Verification items for the finished model (mm, model axes). Coordinates: 2 decimals unless noted, no trailing zeros. Use CSV: the item, a comma, the result in double quotes. Start each with the question number.
```python
from build123d import *

# Parameters (mm, degrees)
BOSS_EXTRUDE2_DEPTH = 9.5
FILLET1_R           = 0.5


with BuildPart() as part:
    # Sketch2 → Boss-Extrude2 (new body, symmetric)
    with BuildSketch(Plane(origin=(0, 0, 0), x_dir=(0, 0, -1), z_dir=(1, 0, 0))):
        with BuildLine():
            Line((0, 12), (0, -12))
            ThreePointArc((0, -12), (-5.710285596, -12.497714363), (-11, -10.29))
            ThreePointArc((-11, -10.29), (-9.540341867, 0), (-11, 10.29))
            ThreePointArc((-11, 10.29), (-5.710285596, 12.497714363), (0, 12))
        make_face()
    extrude(amount=BOSS_EXTRUDE2_DEPTH, both=True)

    # Fillet1
    fillet1_edges = [part.edges().sort_by_distance(p)[0] for p in [
        (9.5, 12.497714363, 5.710285596),
        (9.5, 0, 9.540341867),
        (9.5, -12.497714363, 5.710285596),
        (-9.5, 0, 9.540341867),
        (-9.5, 12.497714363, 5.710285596),
        (-9.5, -12.497714363, 5.710285596),
        (0, -10.29, 11),
        (0, 10.29, 11),
        (0, 12, 0),
        (0, -12, 0),
        (9.5, 0, 0),
    ]]
    fillet(fillet1_edges, radius=FILLET1_R)


solid = part.part
```
Q1. Release check for a two-part mould opening along Y. For faces 1 (the cylindrical face through (0.126, 12.485, 5.791)), 2 (the cylindrical face through (0.13, -0.14, 9.54)), 3 (the flat face through (9.5, 0, 5)), 4 (the cylindrical face through (0.13, -12.51, 5.64)) record: released by +Y, released by -Y, zero draft, split by the parting line, or undercut.
Q2. Gauge pin test, flat ends, axial feed: pin 1 (1.5 mm diameter, centred on x = 0.5, y = -7.5, fed in from +Z); pin 2 (1 mm diameter, centred on x = 6.5, z = 8.5, fed in from -Y); pin 3 (3 mm diameter, centred on x = 4, y = -7.5, fed in from +Z). Record the tip position at first contact, or that the pin passes through.
Q3. Scan lines: line 1 along Y through (x, z) = (-1.75, 4); line 2 along Z through (x, y) = (-0.75, 11.25); line 3 along Z through (x, y) = (1, -9.5). Record each from-to range of solid material in increasing order. Write a range as from..to.
Reply:
1,face 1,"released by +Y"
1,face 2,"undercut"
1,face 3,"zero draft"
1,face 4,"released by -Y"
2,pin 1,"z = 10.47"
2,pin 2,"y = -11.91"
2,pin 3,"z = 10.65"
3,line 1,"-12.64..12.64"
3,line 2,"0..9.47"
3,line 3,"0..10.78"
